from build123d import *

# Parameters (mm, degrees)
SKETCH_R              = 50
SKETCH_R_2            = 25
PAD_DEPTH             = 10
SKETCH001_R           = 10
PAD001_DEPTH          = 10
POLARPATTERN_COUNT    = 5
SKETCH002_R           = 5
SKETCH002_R_2         = 10
POCKET_DEPTH          = 329.680222
POLARPATTERN001_COUNT = 5


with BuildPart() as part:
    # Sketch → Pad (new body)
    with BuildSketch(Plane.XY):
        Circle(SKETCH_R)
        Circle(SKETCH_R_2, mode=Mode.SUBTRACT)
    extrude(amount=PAD_DEPTH)

    # Sketch001 → Pad001 (join)
    with BuildSketch(Plane.XY):
        with Locations((0, 50)):
            Circle(SKETCH001_R)
    pad001 = extrude(amount=PAD001_DEPTH)

    # PolarPattern: Pad001 ×5 about axis
    polarpattern_axis = Axis((0, 0, 0), (0, 0, 1))
    for i in range(1, POLARPATTERN_COUNT):
        add(pad001.rotate(polarpattern_axis, i * 360 / POLARPATTERN_COUNT))

    # Sketch002 (on Face9 of PolarPattern) → Pocket (cut, through all)
    with BuildSketch(Plane.XY.offset(10)):
        with Locations((-1e-06, 50)):
            Circle(SKETCH002_R)
        with Locations((-6e-05, -50)):
            Circle(SKETCH002_R_2)
    pocket = extrude(amount=-POCKET_DEPTH, mode=Mode.SUBTRACT)

    # PolarPattern001: Pocket ×5 about axis
    polarpattern001_axis = Axis((0, 0, 10), (0, 0, 1))
    for i in range(1, POLARPATTERN001_COUNT):
        add(pocket.rotate(polarpattern001_axis, i * 360 / POLARPATTERN001_COUNT), mode=Mode.SUBTRACT)


solid = part.part
Build history of the part. All positions in model axes, mm. A direction names the side the tool comes from. Give positions to 0.01 mm unless a question says otherwise; leave off trailing zeros. Loops run counter-clockwise (first coordinate to the right, second up) from the corner with the lowest first, then second, coordinate; pieces in that order, holes last. Notation, with made-up numbers: (-13, 35) - (33, 35) arc R25 cw to (33, 47) - close; hole circle Ø3 at (-5.75, -5). An arc over 180 degrees is marked (long way). Write item = value, one per line. Start each with the question number.
1) Probe probe 1 along Y at (x, z) = (0, 5.75); probe 2 along X at (y, z) = (-1, 2); probe 3 along Y at (x, z) = (-3, 6). List the from-to ranges inside material, lowest first. Write a range as from..to.
2) Band-saw the part on B-B on y = 0. Give the cut face in (x, z), plus the area to 3 significant figures.
3) Tool access for faces 4 (the cylindrical face through (-35.455, -48.401, 4.93)), 5 (the cylindrical face through (-15.527, -47.528, 4.93)), 6 (the cylindrical face through (40.404, -29.454, 4.93)): list every direction of +Z, -Z, +X, -X, +Y, -Y with a clear straight run to the whole face (end or side of a thin tool).
4) Drop flat-ended pins along their axis: pin 1 Ø6 at (x, y) = (-5.5, 28) entering from -Z; pin 2 Ø1.5 at (x, z) = (22, 6.5) entering from -Y; pin 3 Ø6 at (y, z) = (30, 8.5) entering from +X; pin 4 Ø3 at (x, z) = (11.5, 2.5) entering from -Y. Give the stop position or say it passes through.
5) Pull direction X, two halves, no side cores. Call faces 1 (the flat face through (13, -22, 10)), 2 (the cylindrical face through (-0.651, 54.957, 5.07)), 3 (the cylindrical face through (-50, 0, 5)): +X half, -X half, draft (parallel to the pull), parting line (faces both ways), or undercut.
6) Band-saw the part on D-D on x = -48. Give the cut face in (y, z), plus the area to 3 significant figures.
7) Band-saw the part on C-C on z = 4.5. Give the cut face in (x, y), plus the area to 3 significant figures.
8) Band-saw the part on A-A on x = 0. Give the cut face in (y, z).
Final values:
q1.probe_1 = -40..-25, 25..45, 55..60
q1.probe_2 = -49.99..-24.98, 24.98..49.99
q1.probe_3 = -40.46..-24.82, 24.82..46, 54..59.54
q2.outline = (-50, 0) - (-25, 0) - (-25, 10) - (-50, 10) - close; (25, 0) - (50, 0) - (50, 10) - (25, 10) - close
q2.area = 500 mm²
q3.face_4 = +Z, -Z
q3.face_5 = +Z, -Z, -Y
q3.face_6 = +Z, -Z, +X
q4.pin_1 = 0
q4.pin_2 = -47.93
q4.pin_3 = 42.08
q4.pin_4 = -48.99
q5.face_1 = draft
q5.face_2 = undercut
q5.face_3 = -X half
q6.outline = (-5.46, 0) - (10.47, 0) - (10.47, 10) - (-5.46, 10) - close; (20.43, 0) - (25.44, 0) - (25.44, 10) - (20.43, 10) - close
q6.area = 209 mm²
q7.outline = (-49.68, -5.68) arc R10 cw to (-43.53, -24.6) arc R50 ccw to (-36.85, -33.79) arc R10 ccw (long way) to (-20.75, -45.49) arc R50 ccw to (-9.95, -49) arc R10 cw to (9.95, -49) arc R50 ccw to (20.75, -45.49) arc R10 ccw (long way) to (36.85, -33.79) arc R50 ccw to (43.53, -24.6) arc R10 cw to (49.68, -5.68) arc R50 ccw to (49.68, 5.68) arc R10 ccw (long way) to (43.53, 24.6) arc R50 ccw to (36.85, 33.79) arc R10 cw to (20.75, 45.49) arc R50 ccw to (9.95, 49) arc R10 ccw (long way) to (-9.95, 49) arc R50 ccw to (-20.75, 45.49) arc R10 cw to (-36.85, 33.79) arc R50 ccw to (-43.53, 24.6) arc R10 ccw (long way) to (-49.68, 5.68) arc R50 ccw to start; hole circle Ø10 at (-47.55, 15.45); hole circle Ø10 at (-29.39, -40.45); hole circle Ø50 at (0, 0); hole circle Ø10 at (0, 50); hole circle Ø10 at (29.39, -40.45); hole circle Ø10 at (47.55, 15.45)
q7.area = 5,560 mm²
q8.outline = (-40, 0) - (-25, 0) - (-25, 10) - (-40, 10) - close; (25, 0) - (45, 0) - (45, 10) - (25, 10) - close; (55, 0) - (60, 0) - (60, 10) - (55, 10) - close
